from build123d import *

# Parameters (mm, degrees)
F0_W     = 45
F0_H     = 15
F0_R     = 2.05
F0_R_2   = 0.85
F1_DEPTH = 10
F2_SIZE  = 1.5


with BuildPart() as f1:
    # F0 (on Top) → F1 (new body)
    with BuildSketch(Plane.XY):
        with Locations((12.5, 0)):
            Rectangle(F0_W, F0_H)
        with Locations((-6, 0)):
            Circle(F0_R, mode=Mode.SUBTRACT)
        Circle(F0_R_2, mode=Mode.SUBTRACT)
        with Locations((2.54, 0)):
            Circle(F0_R_2, mode=Mode.SUBTRACT)
        with Locations((5.08, 0)):
            Circle(F0_R_2, mode=Mode.SUBTRACT)
        with Locations((7.62, 0)):
            Circle(F0_R_2, mode=Mode.SUBTRACT)
        with Locations((10.16, 0)):
            Circle(F0_R_2, mode=Mode.SUBTRACT)
        with Locations((12.7, 0)):
            Circle(F0_R_2, mode=Mode.SUBTRACT)
        with Locations((15.24, 0)):
            Circle(F0_R_2, mode=Mode.SUBTRACT)
        with Locations((17.78, 0)):
            Circle(F0_R_2, mode=Mode.SUBTRACT)
        with Locations((20.32, 0)):
            Circle(F0_R_2, mode=Mode.SUBTRACT)
        with Locations((22.86, 0)):
            Circle(F0_R_2, mode=Mode.SUBTRACT)
        with Locations((31, 0)):
            Circle(F0_R, mode=Mode.SUBTRACT)
    extrude(amount=F1_DEPTH)

    # F2
    f2_edges = [f1.edges().sort_by_distance(p)[0] for p in [
        (-8.05, 0, 10),
        (28.95, 0, 10),
    ]]
    chamfer(f2_edges, length=F2_SIZE)


solid = f1.part
Input: part model. Units: mm. Frame: model coordinates. Coordinates: 2 decimals unless noted, no trailing zeros. Loops run counter-clockwise (first coordinate to the right, second up) from the corner with the lowest first, then second, coordinate; pieces in that order, holes last.
Q1. Contact query for a flat-ended pin moving along its axis: pin 1 (2 mm diameter, centred on x = 0, y = 0, fed in from -Z). Output: stop coordinate, or through.
Q2. Cut plane C-C (x = 31). Output: boundary loops of the cut face in (y, z).
Q3. Draft query along Y for faces 1 (the face through (9.31, 0.04, 4.93)), 2 (the face through (12, 2, 0)), 3 (the face through (12, -7.5, 5)), 4 (the face through (13.485, -0.326, 4.93)). Return one class per face: +Y half, -Y half, draft (parallel to the pull), parting line (faces both ways), or undercut.
Q4. Material intervals for line 1 (Y direction, x = 12.7, z = 3); line 2 (Y direction, x = 18.5, z = 2.5); line 3 (Z direction, x = -7, y = -2.75), sorted ascending.
Q5. Cut plane B-B (x = 15.24). Output: boundary loops of the cut face in (y, z).
Q6. Cut plane A-A (z = 5.5). Give the number of separate pieces and of enclosed holes in the cut face, then the cut area to 3 significant figures.
Working result:
1. pin 1: stops at z = 0
2. outline: (-7.5, 0) - (-2.05, 0) - (-2.05, 8.5) - (-3.55, 10) - (-7.5, 10) - close; (2.05, 0) - (7.5, 0) - (7.5, 10) - (3.55, 10) - (2.05, 8.5) - close
3. face 1: undercut
3. face 2: draft
3. face 3: -Y half
3. face 4: undercut
4. line 1: y = -7.5 to -0.85, 0.85 to 7.5
4. line 2: y = -7.5 to -0.45, 0.45 to 7.5
4. line 3: z = 0 to 9.38
5. outline: (-7.5, 0) - (-0.85, 0) - (-0.85, 10) - (-7.5, 10) - close; (0.85, 0) - (7.5, 0) - (7.5, 10) - (0.85, 10) - close
6. separate pieces: 1
6. enclosed holes: 12
6. area: 626 mm2
